Autodesk Inventor part; units mm, degrees
ref_plane "Work Plane1" through (0, 6.35, 0) normal (0, 1, 0) x (1, 0, 0)
ref_plane "YZ Plane" through (0, 0, 0) normal (1, 0, 0) x (0, 1, 0)
ref_plane "XZ Plane" through (0, 0, 0) normal (0, 1, 0) x (-1, 0, 0)
sketch "Sketch1" plane through (0, 0, 0) normal (0, 1, 0) x (-1, 0, 0)
  circle A0 centre (254, -50.8) radius 14.2875
  arc A1 (38.4735, -38.1055) -> (38.4735, -63.4945) centre (38.1, -50.8) ccw
  line L0 (280.9875, -50.8) -> (280.9875, 0)
  line L1 (280.9875, 0) -> (280.9875, -50.8)
  line L2 (280.9875, 0) -> (38.1, 0)
  line L3 (38.1, -38.1) -> (38.1, 0)
  arc A2 (38.4735, -63.4945) -> (43.8871, -100.4525) centre (254, -50.8) ccw
  arc A3 (51.1687, -124.7749) -> (66.9545, -158.6276) centre (254, -50.8) ccw
  arc A4 (80.906, -179.8398) -> (105.7377, -207.743) centre (254, -50.8) ccw
  arc A5 (273.4803, -69.4773) -> (280.9875, -50.8) centre (254, -50.8) ccw
  line L4 (125.2338, -224.0976) -> (273.4803, -69.4773)
  line L5 (280.9875, 0) -> (38.1, 0)
  line L6 (38.1, 0) -> (38.1, -38.1)
  line L7 (280.9875, 0) -> (280.9875, -50.8)
  circle A6 centre (47.1701, -112.7208) radius 6.35
  circle A7 centre (38.1, -50.8) radius 6.35
  arc A8 (43.8871, -100.4525) -> (51.1687, -124.7749) centre (47.1701, -112.7208) ccw
  arc A9 (38.4735, -38.1055) -> (38.4735, -63.4945) centre (38.1, -50.8) ccw
  arc A10 (43.8871, -100.4525) -> (51.1687, -124.7749) centre (47.1701, -112.7208) ccw
  line L8 (38.1, 0) -> (50.8, 0)
  line L9 (38.4739, -38.1) -> (38.1, -38.1)
  line L10 (38.1, -38.1) -> (38.1, 0)
  circle A11 centre (254, -50.8) radius 14.2875
  circle A12 centre (47.1701, -112.7208) radius 6.35
  circle A13 centre (38.1, -50.8) radius 6.35
  arc A14 (51.1687, -124.7749) -> (125.2338, -224.0976) centre (254, -50.8) ccw
  arc A15 (38.1934, -57.1493) -> (43.8871, -100.4525) centre (254, -50.8) ccw
  arc A16 (35.0036, -116.3632) -> (116.3789, -233.3332) centre (254, -50.8) ccw
  line L11 (125.2338, -224.0976) -> (116.3789, -233.3332)
  point P0 (0, 0)
  point P1 (44.1616, 0)
  point P2 (38.1934, -44.4507)
  dimension "d4" = 28.575
  dimension "d32" = 25.4
  dimension "d36" = 50.8
  dimension "d74" = 53.975
  dimension "d79" = 12.7
  dimension "d83" = 26.9875
ref_plane "Work Plane1" through (0, 6.35, 0) normal (0, 1, 0) x (1, 0, 0)
extrude "Extrusion7" add sketch "Sketch1" along normal blind 6.35
sketch "Sketch3" plane through (0, 0, 0) normal (0, -1, 0) x (1, 0, 0)
  circle A0 centre (-254, -50.8) radius 14.2875
  circle A1 centre (-254, -50.8) radius 14.2875
  arc A2 (-116.3789, -233.3332) -> (-35.0036, -116.3632) centre (-254, -50.8) ccw
  circle A3 centre (-47.1701, -112.7208) radius 6.35
  arc A4 (-130.7722, -218.3211) -> (-55.5923, -113.1119) centre (-254, -50.8) ccw
  circle A5 centre (-254, -50.8) radius 24.789
  arc A6 (-126.3412, -222.9426) -> (-47.018, -106.3726) centre (-254, -50.8) ccw
  arc A7 (-54.9513, -130.2322) -> (-60.849, -127.8786) centre (-57.9002, -129.0554) ccw
  line L0 (-62.5231, -105.8831) -> (-35.6006, -133.9631)
  line L1 (-116.3789, -233.3332) -> (-273.4803, -69.4773)
  arc A8 (-120.5628, -210.3083) -> (-116.4883, -215.1788) centre (-118.5256, -212.7436) ccw
  arc A9 (-56.7456, -126.0977) -> (-50.5804, -107.3643) centre (-254, -50.8) ccw
  arc A10 (-128.5564, -220.6321) -> (-120.976, -214.7624) centre (-254, -50.8) ccw
  point P0 (0, 0)
  dimension "d90" = 415.925
  dimension "d94" = 428.625
  dimension "d97" = 6.35
  dimension "d98" = 6.35
  dimension "d101" = 12.7
  dimension "d102" = 6.35
  dimension "d103" = 12.7
extrude "Extrusion8" cut sketch "Sketch3" against normal blind 127 contours A8 A4 A7 A6
sketch "Sketch7" plane through (0, 0, 0) normal (0, -1, 0) x (1, 0, 0)
  line L0 (-280.9875, 0) -> (-38.1, 0)
  line L1 (-217.4875, 0) -> (-369.8875, 0)
  line L2 (-369.8875, 0) -> (-369.8875, -101.6)
  line L3 (-369.8875, -101.6) -> (-217.4875, -101.6)
  line L4 (-217.4875, -101.6) -> (-217.4875, 0)
  line L5 (-280.9875, -50.8) -> (-280.9875, 0)
  line L6 (-116.3789, -233.3332) -> (-273.4803, -69.4773)
  line L7 (-242.6818, -101.6) -> (-276.2977, -52.4082)
  line L8 (-276.2977, -52.4082) -> (-253.5984, 0)
  circle A0 centre (-254, -50.8) radius 14.2875
  circle A1 centre (-254, -50.8) radius 14.2875
  line L9 (-280.9875, 0) -> (-217.4875, 0)
  line L10 (-217.4875, 0) -> (-217.4875, 104.2647)
  line L11 (-217.4875, 104.2647) -> (-280.9875, 104.2647)
  line L12 (-280.9875, 104.2647) -> (-280.9875, 0)
  circle A2 centre (-254, -50.8) radius 76.2
  circle A3 centre (-47.1701, -112.7208) radius 6.35
  line L13 (-254, -50.8) -> (-71.9918, -151.4053)
  arc A4 (-120.5628, -210.3083) -> (-60.849, -127.8786) centre (-254, -50.8) ccw
  point P0 (0, 0)
  dimension "d111" = 63.5
  dimension "d112" = 101.6
  dimension "d113" = 152.4
  dimension "d114" = 115.8875
  dimension "d115" = 152.4
  dimension "d118" = 207.9625
sketch "Sketch8" plane through (0, 0, 0) normal (0, -1, 0) x (1, 0, 0)
  point P0 (0, 0)
properties part number "Hood panel RIGHT" material "Aluminum 6061"
Could you check a few things on this model? Use its own coordinates, in mm. A direction names the side the tool comes from. Coordinates: 2 decimals unless noted, no trailing zeros. Order: outer loops, then holes, each group sorted by start corner. A loop starts at its lowest first (then second) coordinate and runs counter-clockwise, first axis right, second up. Notation, with made-up numbers: (82.25, 41.5) - (139.25, 41.5) arc R25 ccw to (139.25, 68.5) - close; hole circle Ø8 at (83, -29). An arc over 180 degrees is marked (long way). Answer in a Markdown table with one row per item. Add a question column.
(1) Will these pins go through, and if not, where does the flat tip stop? pin 1 (12 mm diameter, centred on x = -55.5, z = -80.5, fed in from -Y); pin 2 (1.5 mm diameter, centred on y = 2, z = -151, fed in from +X); pin 3 (1 mm diameter, centred on y = 3, z = -132, fed in from +X).
(2) If we mould it in two halves opening along Z, with no side actions, what happens to faces 1 (the face through (-279.094, 3.131, -60.731)), 2 (the face through (-56.659, 3.131, -126.133)), 3 (the face through (-151, 6.35, -89))? For each: released by +Z, released by -Z, zero draft, split by the parting line, or undercut.
(3) If we section it at C-C, the plane x = -254: Please give me the cut outline in (y, z), then the cut area to 3 significant figures.
(4) On a 3-axis mill with a long thin cutter (end or side, diameter ignored), from which of +Z, -Z, +X, -X, +Y, -Y can I reach the whole of each face in a straight line? I mean faces 4 (the face through (-38.1, 3, -19)), 5 (the face through (-280.988, 3, -26)), 6 (the face through (-86.01, 3.13, -173.39)), 7 (the face through (-40.418, 3.131, -82.35)). Say none if no direction works.
(5) I need wall thicknesses on L1, parallel to X at y = 2.75, z = -52; L2, parallel to X at y = 4.75, z = -176; L3, parallel to Z at x = -83, y = 1.5. Which ranges of each line are inside material? Lowest first, please.
(6) If we section it at A-A, the plane z = -166.5: Please give me the cut outline in (x, y).
(7) If we section it at D-D, the plane x = -186: Please give me the cut outline in (y, z), then the cut area to 3 significant figures.
(8) If we section it at B-B, the plane y = 2.75: State how many separate pieces and enclosed holes the cut face has, then the cut area to 3 significant figures.
Results are:
| question | item | result |
|---|---|---|
| 1 | pin 1 | stops at y = 0 |
| 1 | pin 2 | stops at x = -48.17 |
| 1 | pin 3 | stops at x = -40.12 |
| 2 | face 1 | released by -Z |
| 2 | face 2 | undercut |
| 2 | face 3 | zero draft |
| 3 | outline | (0, -89.8) - (6.35, -89.8) - (6.35, -65.09) - (0, -65.09) - close; (0, -36.51) - (6.35, -36.51) - (6.35, 0) - (0, 0) - close |
| 3 | area | 389 mm2 |
| 4 | face 4 | +Z, +X, +Y, -Y |
| 4 | face 5 | +Z, -Z, -X, +Y, -Y |
| 4 | face 6 | +Y, -Y |
| 4 | face 7 | +X, +Y, -Y |
| 5 | L1 | x = -280.96 to -268.24, -239.76 to -44.34, -31.86 to -25.46 |
| 5 | L2 | x = -171.35 to -87.95, -80.06 to -62.73 |
| 5 | L3 | z = -202.51 to -179.99, -169.15 to 0 |
| 6 | outline | (-180.46, 0) - (-81.19, 0) - (-81.19, 6.35) - (-180.46, 6.35) - close; (-73.6, 0) - (-56.84, 0) - (-56.84, 6.35) - (-73.6, 6.35) - close |
| 7 | outline | (0, -160.72) - (6.35, -160.72) - (6.35, 0) - (0, 0) - close |
| 7 | area | 1,020 mm2 |
| 8 | separate pieces | 1 |
| 8 | enclosed holes | 4 |
| 8 | area | 37,800 mm2 |
